Autodesk Inventor part; units mm, degrees
ref_plane "YZ Plane" through (0, 0, 0) normal (1, 0, 0) x (0, 1, 0)
ref_plane "XZ Plane" through (0, 0, 0) normal (0, 1, 0) x (-1, 0, 0)
ref_plane "XY Plane" through (0, 0, 0) normal (0, 0, 1) x (1, 0, 0)
sketch "Sketch1" plane through (0, 0, 0) normal (0, 1, 0) x (-1, 0, 0)
  line L0 (183.8315, -67.9127) -> (183.8315, 67.9127) construction
  line L1 (-179.8315, 79.4127) -> (-126.5543, 79.4127) construction
  line L2 (-122.5543, 75.4127) -> (-122.5543, 71.9127) construction
  line L3 (-81.7029, 71.9127) -> (-81.7029, 75.4127) construction
  line L4 (-77.7029, 79.4127) -> (-24.4257, 79.4127) construction
  line L5 (-20.4257, 75.4127) -> (-20.4257, 71.9127) construction
  line L6 (20.4257, 71.9127) -> (20.4257, 75.4127) construction
  line L7 (24.4257, 79.4127) -> (77.7029, 79.4127) construction
  line L8 (81.7029, 75.4127) -> (81.7029, 71.9127) construction
  line L9 (122.5543, 71.9127) -> (122.5543, 75.4127) construction
  line L10 (126.5543, 79.4127) -> (179.8315, 79.4127) construction
  line L11 (183.8315, 75.4127) -> (183.8315, 71.9127) construction
  line L12 (-126.5543, -79.4127) -> (-179.8315, -79.4127) construction
  line L13 (-183.8315, -75.4127) -> (-183.8315, -71.9127) construction
  line L14 (-122.5543, -71.9127) -> (-122.5543, -75.4127) construction
  line L15 (-81.7029, -75.4127) -> (-81.7029, -71.9127) construction
  line L16 (-24.4257, -79.4127) -> (-77.7029, -79.4127) construction
  line L17 (-20.4257, -71.9127) -> (-20.4257, -75.4127) construction
  line L18 (20.4257, -75.4127) -> (20.4257, -71.9127) construction
  line L19 (77.7029, -79.4127) -> (24.4257, -79.4127) construction
  line L20 (81.7029, -71.9127) -> (81.7029, -75.4127) construction
  line L21 (122.5543, -75.4127) -> (122.5543, -71.9127) construction
  line L22 (179.8315, -79.4127) -> (126.5543, -79.4127) construction
  line L23 (183.8315, -71.9127) -> (183.8315, -75.4127) construction
  line L24 (-122.5543, -71.9127) -> (-81.7029, -71.9127) construction
  line L25 (-20.4257, -71.9127) -> (20.4257, -71.9127) construction
  line L26 (81.7029, -71.9127) -> (122.5543, -71.9127) construction
  arc A0 (-183.8315, -75.4127) -> (-179.8315, -79.4127) centre (-179.8315, -75.4127) ccw construction
  arc A1 (-126.5543, -79.4127) -> (-122.5543, -75.4127) centre (-126.5543, -75.4127) ccw construction
  arc A2 (-81.7029, -75.4127) -> (-77.7029, -79.4127) centre (-77.7029, -75.4127) ccw construction
  arc A3 (-24.4257, -79.4127) -> (-20.4257, -75.4127) centre (-24.4257, -75.4127) ccw construction
  arc A4 (20.4257, -75.4127) -> (24.4257, -79.4127) centre (24.4257, -75.4127) ccw construction
  arc A5 (77.7029, -79.4127) -> (81.7029, -75.4127) centre (77.7029, -75.4127) ccw construction
  arc A6 (122.5543, -75.4127) -> (126.5543, -79.4127) centre (126.5543, -75.4127) ccw construction
  arc A7 (179.8315, -79.4127) -> (183.8315, -75.4127) centre (179.8315, -75.4127) ccw construction
  line L27 (183.8315, -67.9127) -> (183.8315, -71.9127) construction
  arc A8 (-179.8315, 79.4127) -> (-183.8315, 75.4127) centre (-179.8315, 75.4127) ccw construction
  arc A9 (-122.5543, 75.4127) -> (-126.5543, 79.4127) centre (-126.5543, 75.4127) ccw construction
  line L28 (-81.7029, 71.9127) -> (-122.5543, 71.9127) construction
  line L29 (20.4257, 71.9127) -> (-20.4257, 71.9127) construction
  line L30 (122.5543, 71.9127) -> (81.7029, 71.9127) construction
  line L31 (183.8315, 71.9127) -> (183.8315, 67.9127) construction
  arc A10 (-77.7029, 79.4127) -> (-81.7029, 75.4127) centre (-77.7029, 75.4127) ccw construction
  arc A11 (-20.4257, 75.4127) -> (-24.4257, 79.4127) centre (-24.4257, 75.4127) ccw construction
  arc A12 (24.4257, 79.4127) -> (20.4257, 75.4127) centre (24.4257, 75.4127) ccw construction
  arc A13 (81.7029, 75.4127) -> (77.7029, 79.4127) centre (77.7029, 75.4127) ccw construction
  arc A14 (126.5543, 79.4127) -> (122.5543, 75.4127) centre (126.5543, 75.4127) ccw construction
  arc A15 (183.8315, 75.4127) -> (179.8315, 79.4127) centre (179.8315, 75.4127) ccw construction
  line L32 (-183.8315, 75.4127) -> (-183.8315, -71.9127) construction
  line L33 (-126.5543, 79.9127) -> (-179.8315, 79.9127)
  arc A16 (-179.8315, 79.9127) -> (-184.3315, 75.4127) centre (-179.8315, 75.4127) ccw
  line L34 (-184.3315, 75.4127) -> (-184.3315, -71.9127)
  line L35 (-184.3315, -71.9127) -> (-184.3315, -75.4127)
  arc A17 (-184.3315, -75.4127) -> (-179.8315, -79.9127) centre (-179.8315, -75.4127) ccw
  line L36 (-179.8315, -79.9127) -> (-126.5543, -79.9127)
  arc A18 (-126.5543, -79.9127) -> (-122.0543, -75.4127) centre (-126.5543, -75.4127) ccw
  line L37 (-122.0543, -75.4127) -> (-122.0543, -72.4127)
  line L38 (-122.0543, -72.4127) -> (-82.2029, -72.4127)
  line L39 (-82.2029, -72.4127) -> (-82.2029, -75.4127)
  arc A19 (-82.2029, -75.4127) -> (-77.7029, -79.9127) centre (-77.7029, -75.4127) ccw
  line L40 (-77.7029, -79.9127) -> (-24.4257, -79.9127)
  arc A20 (-24.4257, -79.9127) -> (-19.9257, -75.4127) centre (-24.4257, -75.4127) ccw
  line L41 (-19.9257, -75.4127) -> (-19.9257, -72.4127)
  line L42 (-19.9257, -72.4127) -> (19.9257, -72.4127)
  line L43 (19.9257, -72.4127) -> (19.9257, -75.4127)
  arc A21 (19.9257, -75.4127) -> (24.4257, -79.9127) centre (24.4257, -75.4127) ccw
  line L44 (24.4257, -79.9127) -> (77.7029, -79.9127)
  arc A22 (77.7029, -79.9127) -> (82.2029, -75.4127) centre (77.7029, -75.4127) ccw
  line L45 (82.2029, -75.4127) -> (82.2029, -72.4127)
  line L46 (82.2029, -72.4127) -> (122.0543, -72.4127)
  line L47 (122.0543, -72.4127) -> (122.0543, -75.4127)
  arc A23 (122.0543, -75.4127) -> (126.5543, -79.9127) centre (126.5543, -75.4127) ccw
  line L48 (126.5543, -79.9127) -> (179.8315, -79.9127)
  arc A24 (179.8315, -79.9127) -> (184.3315, -75.4127) centre (179.8315, -75.4127) ccw
  line L49 (184.3315, -75.4127) -> (184.3315, -71.9127)
  line L50 (184.3315, -71.9127) -> (184.3315, -67.9127)
  line L51 (184.3315, -67.9127) -> (184.3315, 67.9127)
  line L52 (184.3315, 67.9127) -> (184.3315, 71.9127)
  line L53 (184.3315, 71.9127) -> (184.3315, 75.4127)
  arc A25 (184.3315, 75.4127) -> (179.8315, 79.9127) centre (179.8315, 75.4127) ccw
  line L54 (179.8315, 79.9127) -> (126.5543, 79.9127)
  arc A26 (126.5543, 79.9127) -> (122.0543, 75.4127) centre (126.5543, 75.4127) ccw
  line L55 (122.0543, 75.4127) -> (122.0543, 72.4127)
  line L56 (122.0543, 72.4127) -> (82.2029, 72.4127)
  line L57 (82.2029, 72.4127) -> (82.2029, 75.4127)
  arc A27 (82.2029, 75.4127) -> (77.7029, 79.9127) centre (77.7029, 75.4127) ccw
  line L58 (77.7029, 79.9127) -> (24.4257, 79.9127)
  arc A28 (24.4257, 79.9127) -> (19.9257, 75.4127) centre (24.4257, 75.4127) ccw
  line L59 (19.9257, 75.4127) -> (19.9257, 72.4127)
  line L60 (19.9257, 72.4127) -> (-19.9257, 72.4127)
  line L61 (-19.9257, 72.4127) -> (-19.9257, 75.4127)
  arc A29 (-19.9257, 75.4127) -> (-24.4257, 79.9127) centre (-24.4257, 75.4127) ccw
  line L62 (-24.4257, 79.9127) -> (-77.7029, 79.9127)
  arc A30 (-77.7029, 79.9127) -> (-82.2029, 75.4127) centre (-77.7029, 75.4127) ccw
  line L63 (-82.2029, 75.4127) -> (-82.2029, 72.4127)
  line L64 (-82.2029, 72.4127) -> (-122.0543, 72.4127)
  line L65 (-122.0543, 72.4127) -> (-122.0543, 75.4127)
  arc A31 (-122.0543, 75.4127) -> (-126.5543, 79.9127) centre (-126.5543, 75.4127) ccw
  line L66 (-179.8315, 75.4127) -> (179.8315, -75.4127) construction
  line L67 (179.8315, 75.4127) -> (-179.8315, -75.4127) construction
  line L68 (-192.3315, 84.9127) -> (192.3315, 84.9127)
  line L69 (194.3315, 82.9127) -> (194.3315, -82.9127)
  line L70 (192.3315, -84.9127) -> (-192.3315, -84.9127)
  line L71 (-194.3315, -82.9127) -> (-194.3315, 82.9127)
  line L72 (-194.3315, 84.9127) -> (194.3315, -84.9127) construction
  line L73 (194.3315, 84.9127) -> (-194.3315, -84.9127) construction
  arc A32 (-192.3315, 84.9127) -> (-194.3315, 82.9127) centre (-192.3315, 82.9127) ccw
  arc A33 (194.3315, 82.9127) -> (192.3315, 84.9127) centre (192.3315, 82.9127) ccw
  arc A34 (192.3315, -84.9127) -> (194.3315, -82.9127) centre (192.3315, -82.9127) ccw
  arc A35 (-194.3315, -82.9127) -> (-192.3315, -84.9127) centre (-192.3315, -82.9127) ccw
  point P0 (0, 0)
  point P1 (0, 0)
  dimension "d9" = 4
  dimension "d10" = 4
  dimension "d11" = 4
  dimension "d12" = 4
  dimension "d13" = 0.5
  dimension "d16" = 159.8253
  dimension "d17" = 368.6629
  dimension "d18" = 388.6629
  dimension "d19" = 169.8253
  dimension "d20" = 2
extrude "Extrusion1" add sketch "Sketch1" against normal blind 4
sketch "Sketch2" plane through (0, -4, 0) normal (0, -1, 0) x (1, 0, 0)
  line L0 (-192.3315, -84.9127) -> (192.3315, -84.9127)
  arc A0 (192.3315, -84.9127) -> (194.3315, -82.9127) centre (192.3315, -82.9127) ccw
  line L1 (194.3315, -82.9127) -> (194.3315, 82.9127)
  arc A1 (194.3315, 82.9127) -> (192.3315, 84.9127) centre (192.3315, 82.9127) ccw
  line L2 (192.3315, 84.9127) -> (-192.3315, 84.9127)
  arc A2 (-192.3315, 84.9127) -> (-194.3315, 82.9127) centre (-192.3315, 82.9127) ccw
  line L3 (-194.3315, 82.9127) -> (-194.3315, -82.9127)
  arc A3 (-194.3315, -82.9127) -> (-192.3315, -84.9127) centre (-192.3315, -82.9127) ccw
  arc A4 (126.5543, 79.9127) -> (122.0543, 75.4127) centre (126.5543, 75.4127) ccw
  line L4 (126.5543, 79.9127) -> (179.8315, 79.9127)
  arc A5 (184.3315, 75.4127) -> (179.8315, 79.9127) centre (179.8315, 75.4127) ccw
  line L5 (184.3315, 75.4127) -> (184.3315, -75.4127)
  arc A6 (179.8315, -79.9127) -> (184.3315, -75.4127) centre (179.8315, -75.4127) ccw
  line L6 (179.8315, -79.9127) -> (126.5543, -79.9127)
  arc A7 (122.0543, -75.4127) -> (126.5543, -79.9127) centre (126.5543, -75.4127) ccw
  line L7 (122.0543, -75.4127) -> (122.0543, -72.4127)
  line L8 (122.0543, -72.4127) -> (82.2029, -72.4127)
  line L9 (82.2029, -72.4127) -> (82.2029, -75.4127)
  arc A8 (77.7029, -79.9127) -> (82.2029, -75.4127) centre (77.7029, -75.4127) ccw
  line L10 (77.7029, -79.9127) -> (24.4257, -79.9127)
  arc A9 (19.9257, -75.4127) -> (24.4257, -79.9127) centre (24.4257, -75.4127) ccw
  line L11 (19.9257, -75.4127) -> (19.9257, -72.4127)
  line L12 (19.9257, -72.4127) -> (-19.9257, -72.4127)
  line L13 (-19.9257, -72.4127) -> (-19.9257, -75.4127)
  arc A10 (-24.4257, -79.9127) -> (-19.9257, -75.4127) centre (-24.4257, -75.4127) ccw
  line L14 (-24.4257, -79.9127) -> (-77.7029, -79.9127)
  arc A11 (-82.2029, -75.4127) -> (-77.7029, -79.9127) centre (-77.7029, -75.4127) ccw
  line L15 (-82.2029, -75.4127) -> (-82.2029, -72.4127)
  line L16 (-82.2029, -72.4127) -> (-122.0543, -72.4127)
  line L17 (-122.0543, -72.4127) -> (-122.0543, -75.4127)
  arc A12 (-126.5543, -79.9127) -> (-122.0543, -75.4127) centre (-126.5543, -75.4127) ccw
  line L18 (-126.5543, -79.9127) -> (-179.8315, -79.9127)
  arc A13 (-184.3315, -75.4127) -> (-179.8315, -79.9127) centre (-179.8315, -75.4127) ccw
  line L19 (-184.3315, -75.4127) -> (-184.3315, 75.4127)
  arc A14 (-179.8315, 79.9127) -> (-184.3315, 75.4127) centre (-179.8315, 75.4127) ccw
  line L20 (-179.8315, 79.9127) -> (-126.5543, 79.9127)
  arc A15 (-122.0543, 75.4127) -> (-126.5543, 79.9127) centre (-126.5543, 75.4127) ccw
  line L21 (-122.0543, 75.4127) -> (-122.0543, 72.4127)
  line L22 (-122.0543, 72.4127) -> (-82.2029, 72.4127)
  line L23 (-82.2029, 72.4127) -> (-82.2029, 75.4127)
  arc A16 (-77.7029, 79.9127) -> (-82.2029, 75.4127) centre (-77.7029, 75.4127) ccw
  line L24 (-77.7029, 79.9127) -> (-24.4257, 79.9127)
  arc A17 (-19.9257, 75.4127) -> (-24.4257, 79.9127) centre (-24.4257, 75.4127) ccw
  line L25 (-19.9257, 75.4127) -> (-19.9257, 72.4127)
  line L26 (-19.9257, 72.4127) -> (19.9257, 72.4127)
  line L27 (19.9257, 72.4127) -> (19.9257, 75.4127)
  arc A18 (24.4257, 79.9127) -> (19.9257, 75.4127) centre (24.4257, 75.4127) ccw
  line L28 (24.4257, 79.9127) -> (77.7029, 79.9127)
  arc A19 (82.2029, 75.4127) -> (77.7029, 79.9127) centre (77.7029, 75.4127) ccw
  line L29 (82.2029, 75.4127) -> (82.2029, 72.4127)
  line L30 (82.2029, 72.4127) -> (122.0543, 72.4127)
  line L31 (122.0543, 72.4127) -> (122.0543, 75.4127)
  line L32 (-184.3315, -75.4127) -> (-184.3315, 75.4127)
  line L33 (184.3315, 75.4127) -> (184.3315, -75.4127)
  line L34 (-184.3315, 72.4127) -> (184.3315, 72.4127)
  line L35 (184.3315, 72.4127) -> (184.3315, -72.4127)
  line L36 (184.3315, -72.4127) -> (-184.3315, -72.4127)
  line L37 (-184.3315, -72.4127) -> (-184.3315, 72.4127)
  point P0 (0, 0)
extrude "Extrusion2" add sketch "Sketch2" along normal blind 7 contours A3 L3 A2 L2 A1 L1 A0 L0 | L4 A5 L5 L34 L31 A4 | L34 L27 A18 L28 A19 L29 | L5 A6 L6 A7 L7 L36 | L34 L23 A16 L24 A17 L25 | L9 A8 L10 A9 L11 L36 | L34 L19 A14 L20 A15 L21 | L13 A10 L14 A11 L15 L36 | L36 L17 A12 L18 A13 L19
sketch "Sketch3" plane through (0, -11, 0) normal (0, -1, 0) x (1, 0, 0)
  arc A0 (192.3315, -84.9127) -> (194.3315, -82.9127) centre (192.3315, -82.9127) ccw
  line L0 (194.3315, -82.9127) -> (194.3315, 82.9127)
  arc A1 (194.3315, 82.9127) -> (192.3315, 84.9127) centre (192.3315, 82.9127) ccw
  line L1 (192.3315, 84.9127) -> (-192.3315, 84.9127)
  arc A2 (-192.3315, 84.9127) -> (-194.3315, 82.9127) centre (-192.3315, 82.9127) ccw
  line L2 (-194.3315, 82.9127) -> (-194.3315, -82.9127)
  arc A3 (-194.3315, -82.9127) -> (-192.3315, -84.9127) centre (-192.3315, -82.9127) ccw
  line L3 (-192.3315, -84.9127) -> (192.3315, -84.9127)
  line L4 (184.3315, 72.4127) -> (184.3315, -72.4127)
  line L5 (184.3315, -72.4127) -> (-184.3315, -72.4127)
  line L6 (-184.3315, -72.4127) -> (-184.3315, 72.4127)
  line L7 (-184.3315, 72.4127) -> (184.3315, 72.4127)
  point P0 (0, 0)
extrude "Extrusion3" add sketch "Sketch3" along normal blind 7 contours L3 A3 L2 A2 L1 A1 L0 A0 | L4 L5 L6 L7
properties part number "kbbottombodyethan"
Input: part model. Units: mm. Frame: model coordinates. A direction names the side the tool comes from. Round coordinates to 2 decimals unless told otherwise and drop trailing zeros. Write each loop counter-clockwise with the first axis right and the second up, starting at its lowest first coordinate (ties: lowest second). Pieces come first, ordered by that corner, then holes. Notation, with made-up numbers: M -14,86.5 L 14,86.5 A27 cw 14,103.5 Z; hole C 80,-4 d1. An arc over 180 degrees is marked long. Write each question's results on one line, items separated by ' | '.
Q1. Pin query (flat end, axial travel): P1, Ø8, axis at x = -161.5, z = -74.5, coming from the +Y side. Return the tip coordinate at first contact, or that it passes through.
Results:
P1: stops at y = -4
Q2. Access query for faces 4 (the face through (1, 0, 76)), 5 (the face through (-3, -7, 72.413)). Directions: +Z, -Z, +X, -X, +Y, -Y. A direction counts if a zero-diameter tool reaches every point of the face in a straight line with its end or side. Return the directions, or none.
Results:
face 4: +Z, -Z, +X, -X, +Y | face 5: +Y
Q3. Section query D-D (x = -154.5). Return loops of the section in (y, z).
Results:
outline: M -18,-84.91 L 0,-84.91 L 0,-79.91 L -4,-79.91 L -4,-72.41 L -11,-72.41 L -11,72.41 L -4,72.41 L -4,79.91 L 0,79.91 L 0,84.91 L -18,84.91 Z
Q4. Draft query along X for faces 1 (the face through (153, -4, 76)), 2 (the face through (3, -9, 84.913)), 3 (the face through (-194.332, -9, 1)). Return one class per face: released by +X, released by -X, zero draft, split by the parting line, or undercut.
Results:
face 1: undercut | face 2: zero draft | face 3: released by -X
Q5. Section query C-C (x = -107). Return loops of the section in (y, z), and give its area (3 significant figures).
Results:
outline: M -18,-84.91 L 0,-84.91 L 0,-72.41 L -11,-72.41 L -11,72.41 L 0,72.41 L 0,84.91 L -18,84.91 Z | area: 1,460 mm^2
Q6. Section query B-B (z = 51.5). Return loops of the section in (x, y).
Results:
outline: M -194.33,-18 L 194.33,-18 L 194.33,0 L 184.33,0 L 184.33,-11 L -184.33,-11 L -184.33,0 L -194.33,0 Z
Q7. Section query A-A (y = -8). Return loops of the section in (x, z).
Results:
outline: M -194.33,-82.91 A2 ccw -192.33,-84.91 L 192.33,-84.91 A2 ccw 194.33,-82.91 L 194.33,82.91 A2 ccw 192.33,84.91 L -192.33,84.91 A2 ccw -194.33,82.91 Z; hole M -184.33,-72.41 L 184.33,-72.41 L 184.33,72.41 L -184.33,72.41 Z
Q8. Line query: line 1 along X through (y, z) = (-4.25, -64); line 2 along Z through (x, y) = (-99.5, -7.25); line 3 along Z through (x, y) = (-177, -2.5). Output: solid intervals per line, ascending.
Results:
line 1: x = -194.33 to -184.33, 184.33 to 194.33 | line 2: z = -84.91 to -72.41, 72.41 to 84.91 | line 3: z = -84.91 to -79.91, 79.91 to 84.91
